```python
from build123d import *

# Parameters (mm, degrees)
BOSS_EXTRUDE1_DEPTH = 2
FILLET2_R           = 1
CHAMFER1_SIZE       = 0.8
SKETCH4_R           = 6.925
SKETCH4_R_2         = 4.6
BOSS_EXTRUDE2_DEPTH = 3


with BuildPart() as part:
    # Sketch2 → Revolve1 (revolve)
    with BuildSketch(Plane(origin=(0, 0, 0), x_dir=(1, 0, 0), z_dir=(0, 1, 0))):
        Polygon((-3.5, -12.32), (-3.5, -11.68), (-4.925, -11.2), (-4.925, -8.7), (-3.45, -8.7), (-3.45, -7.5), (-5, -7.5), (-5, 0), (-13.4, 0), (-13.4, -2), (-6.925, -2), (-6.925, -12.32), align=None)
    revolve(axis=Axis((0, 0, 0), (0, 0, 1)))

    # Sketch3 → Boss-Extrude1 (add)
    with BuildSketch(Plane.XY.offset(2)):
        with BuildLine():
            Line((10, 8.919641248), (10, 25.121576202))
            Line((10, 25.121576202), (-10, 25.121576202))
            Line((-10, 25.121576202), (-10, 8.919641248))
            ThreePointArc((-10, 8.919641248), (0, 13.4), (10, 8.919641248))
        make_face()
    extrude(amount=-BOSS_EXTRUDE1_DEPTH)

    # Fillet2
    fillet2_edges = [part.edges().sort_by_distance(p)[0] for p in [
        (10, 25.121576202, 1),
        (-10, 25.121576202, 1),
        (-10, 8.919641248, 1),
        (10, 8.919641248, 1),
    ]]
    fillet(fillet2_edges, radius=FILLET2_R)

    # Chamfer1
    chamfer1_edges = [part.edges().sort_by_distance(p)[0] for p in [
        (6.925, 0, 2),
    ]]
    chamfer(chamfer1_edges, length=CHAMFER1_SIZE)

    # Sketch4 → Boss-Extrude2 (add)
    with BuildSketch(Plane.XY.offset(12.32)):
        with Locations(Location((0, 0, 0), (0, 0, 180))):
            Circle(SKETCH4_R)
        Circle(SKETCH4_R_2, mode=Mode.SUBTRACT)
    extrude(amount=BOSS_EXTRUDE2_DEPTH)


solid = part.part
```
Work out the finished part from the listing and answer in its coordinate system (mm). A direction names the side the tool comes from. Give positions to 0.01 mm unless a question says otherwise; leave off trailing zeros. Write each loop counter-clockwise with the first axis right and the second up, starting at its lowest first coordinate (ties: lowest second). Pieces come first, ordered by that corner, then holes. Notation, with made-up numbers: (6, -27.5) - (47, -27.5) arc R17 cw to (47, 3.5) - close; hole circle Ø8 at (34.25, -13). An arc over 180 degrees is marked (long way). Use one line per item in the form item = value.
1. For faces 1 (the face through (3.908, 2.997, 9.932)), 2 (the face through (-10, 17, 1)), 3 (the face through (0, 10, 2)), determine the directions among +Z, -Z, +X, -X, +Y, -Y from which every point of the face is accessible in a straight line to the end or side of a thin tool.
Filled in:
face_1 = none
face_2 = +Z, -Z, -X, +Y
face_3 = +Z
2. Consider L1, parallel to Y at x = 0, z = 14.45 (3 decimals); L2, parallel to Y at x = 0, z = 12.15 (3 decimals); L3, parallel to Z at x = -9.75, y = 17.5. Determine where each line is inside the solid, lowest interval first.
Filled in:
L1 = -6.925 to -4.6, 4.6 to 6.925
L2 = -6.925 to -3.5, 3.5 to 6.925
L3 = 0 to 2
3. A cutting plane is placed at D-D (y = 14). Write down the section's boundary in (x, z), and give its area (3 significant figures).
Filled in:
outline = (-10, 0) - (10, 0) - (10, 2) - (-10, 2) - close
area = 40.0 mm^2
4. A cutting plane is placed at C-C (z = 5). Write down the section's boundary in (x, y) (3 decimals), and give its area (3 significant figures).
Filled in:
outline = circle Ø13.85 at (0, 0); hole circle Ø10 at (0, 0)
area = 72.1 mm^2
5. Each of these flat-tipped pins is pushed along its axis until it touches: pin 1 Ø4.5 at (x, y) = (1.5, 1) entering from +Z; pin 2 Ø1.5 at (x, z) = (-9.5, 13.5) entering from -Y; pin 3 Ø3 at (x, y) = (4, 15) entering from +Z; pin 4 Ø1 at (y, z) = (16, 1) entering from -X. Where does it stop, or does it pass through?
Filled in:
pin_1 = 12.32
pin_2 = through
pin_3 = 2
pin_4 = -10
6. Determine the mould class of faces 4 (the face through (-1.2, -3.4, 7.5)), 5 (the face through (2.41, -2.75, 12.32)), 6 (the face through (1.2, -3.4, 8.7)) for opening direction Z: released by +Z, released by -Z, zero draft, split by the parting line, or undercut.
Filled in:
face_4 = released by -Z
face_5 = released by +Z
face_6 = undercut
